Autodesk Inventor part; units mm, degrees
ref_plane "YZ Plane" through (0, 0, 0) normal (1, 0, 0) x (0, 1, 0)
ref_plane "XZ Plane" through (0, 0, 0) normal (0, 1, 0) x (-1, 0, 0)
ref_plane "XY Plane" through (0, 0, 0) normal (0, 0, 1) x (1, 0, 0)
sketch "Sketch1" plane through (0, 0, 0) normal (0, 0, 1) x (1, 0, 0)
  line L0 (0, 0) -> (25.4, 0)
  line L1 (25.4, 0) -> (25.4, 50.8)
  line L2 (25.4, 50.8) -> (0, 50.8)
  line L3 (0, 50.8) -> (0, 0)
  dimension "d0" = 25.4
  dimension "d1" = 50.8
extrude "Extrusion1" add sketch "Sketch1" along normal blind 203.2
shell "Shell1" thickness 2.54 removed faces 2 at (8.4667, 33.8667, 0) at (8.4667, 33.8667, 203.2)
sketch "Sketch2" plane through (0, 50.8, 0) normal (0, 1, 0) x (1, 0, 0)
  line L0 (25.4, 0) -> (0, 0)
  line L1 (0, 0) -> (0, -203.2)
  point P0 (12.7, -12.7)
  point P1 (12.7, -38.1)
  point P2 (12.7, -63.5)
  point P3 (12.7, -88.9)
  point P4 (12.7, -114.3)
  point P5 (12.7, -139.7)
  point P6 (12.7, -165.1)
  point P7 (12.7, -190.5)
  point P8 (12.7, -215.9)
  point P9 (12.7, -241.3)
  point P10 (12.7, -266.7)
  point P11 (12.7, -292.1)
  point P12 (12.7, -317.5)
  point P13 (12.7, -342.9)
  point P14 (12.7, -368.3)
  point P15 (12.7, -393.7)
  point P16 (12.7, -419.1)
  point P17 (12.7, -444.5)
  point P18 (12.7, -469.9)
  point P19 (12.7, -495.3)
  point P20 (12.7, -520.7)
  point P21 (12.7, -546.1)
  point P22 (12.7, -571.5)
  point P23 (12.7, -596.9)
  point P24 (12.7, -622.3)
  point P25 (12.7, -647.7)
  point P26 (12.7, -673.1)
  point P27 (12.7, -698.5)
  point P28 (12.7, -723.9)
  point P29 (12.7, -749.3)
  point P30 (12.7, -774.7)
  point P31 (12.7, -800.1)
  point P32 (12.7, -825.5)
  point P33 (12.7, -850.9)
  point P34 (12.7, -876.3)
  point P35 (12.7, -901.7)
  point P36 (12.7, -927.1)
  dimension "d5" = 12.7
  dimension "d6" = 12.7
  dimension "d9" = 25.4
hole "Hole1" at (12.7, 50.8, 12.7) at (12.7, 50.8, 38.1) at (12.7, 50.8, 63.5) at (12.7, 50.8, 88.9) at (12.7, 50.8, 114.3) at (12.7, 50.8, 139.7) at (12.7, 50.8, 165.1) at (12.7, 50.8, 190.5) at (12.7, 50.8, 215.9) at (12.7, 50.8, 241.3) at (12.7, 50.8, 266.7) at (12.7, 50.8, 292.1) at (12.7, 50.8, 317.5) at (12.7, 50.8, 342.9) at (12.7, 50.8, 368.3) at (12.7, 50.8, 393.7) at (12.7, 50.8, 419.1) at (12.7, 50.8, 444.5) at (12.7, 50.8, 469.9) at (12.7, 50.8, 495.3) at (12.7, 50.8, 520.7) at (12.7, 50.8, 546.1) at (12.7, 50.8, 571.5) at (12.7, 50.8, 596.9) at (12.7, 50.8, 622.3) at (12.7, 50.8, 647.7) at (12.7, 50.8, 673.1) at (12.7, 50.8, 698.5) at (12.7, 50.8, 723.9) at (12.7, 50.8, 749.3) at (12.7, 50.8, 774.7) at (12.7, 50.8, 800.1) at (12.7, 50.8, 825.5) at (12.7, 50.8, 850.9) at (12.7, 50.8, 876.3) at (12.7, 50.8, 901.7) direction (0, -1, 0) diameter 2.54 depth 50.8 tip angle 118
sketch "Sketch14" plane through (0, 0, 0) normal (-1, 0, 0) x (0, 0, 1)
  circle A0 centre (25.4, 25.4) radius 6.35
  point P0 (0, 0)
hole "Hole6" at (0, 25.4, 25.4) direction (1, 0, 0) diameter 28.575 depth 25.4 tip angle 118
sketch "Sketch15" plane through (25.4, 0, 0) normal (1, 0, 0) x (0, 0, -1)
  circle A0 centre (-177.8, 25.4) radius 20
  point P0 (0, 0)
hole "Hole7" at (25.4, 25.4, 177.8) direction (-1, 0, 0) diameter 28.575 depth 25.4 tip angle 118
sketch "Sketch16" plane through (25.4, 0, 0) normal (1, 0, 0) x (0, 0, -1)
  circle A0 centre (-159.8395, 43.3605) radius 3.3655
  circle A1 centre (-195.7605, 7.4395) radius 3.3655
  circle A2 centre (-195.3, 42.9) radius 3.3655
  circle A3 centre (-160.3, 7.9) radius 3.1115
  point P0 (0, 0)
hole "Hole8" at (25.4, 7.9, 160.3) at (25.4, 43.3605, 159.8395) at (25.4, 42.9, 195.3) at (25.4, 7.4395, 195.7605) direction (-1, 0, 0) diameter 4.4958 depth 25.4 tip angle 118
properties part number "Support Pivs 2522" material "Aluminum 6061"
The listing builds one solid part. Answer for the finished solid, in the listing's coordinates (mm). A direction names the side the tool comes from. Give positions to 0.01 mm unless a question says otherwise; leave off trailing zeros. Order: outer loops, then holes, each group sorted by start corner. A loop starts at its lowest first (then second) coordinate and runs counter-clockwise, first axis right, second up. Notation, with made-up numbers: (-20, 3.5) - (25, 3.5) arc R4 cw to (25, 8.5) - close; hole circle Ø6 at (84, 44.25). An arc over 180 degrees is marked (long way). Use one line per item in the form item = value. Start each with the question number.
(1) A cutting plane is placed at B-B, the plane y = 35.5. Write down the section's boundary in (x, z).
(2) A cutting plane is placed at A-A, the plane x = 7. Write down the section's boundary in (y, z).
(3) Consider line 1 (Z direction, x = 23.5, y = 25.5); line 2 (Y direction, x = 24.25, z = 25.4); line 3 (Y direction, x = 12.25, z = 148.5). Determine where each line is inside the solid, lowest interval first. Write a range as from..to.
(4) The mould has two halves that part along Y. Classify faces 1 (the flat face through (13, 50.8, 100)), 2 (the flat face through (2, 27, 203.2)), 3 (the flat face through (13, 0, 100)), 4 (the cylindrical face through (1.252, 42.225, 193.156)): released by +Y, released by -Y, zero draft, split by the parting line, or undercut.
(5) A cutting plane is placed at D-D, the plane z = 195.3. Write down the section's boundary in (x, y), then the cut area to 3 significant figures.
(6) A cutting plane is placed at C-C, the plane z = 45. Write down the section's boundary in (x, y).
(7) For faces 5 (the cylindrical face through (24.148, 15.744, 14.87)), 6 (the flat face through (22.86, 25, 100)), determine the directions among +Z, -Z, +X, -X, +Y, -Y from which every point of the face is accessible in a straight line to the end or side of a thin tool.
Ans:
q1.outline = (0, 0) - (2.54, 0) - (2.54, 15.29) - (0, 15.29) - close; (0, 35.51) - (2.54, 35.51) - (2.54, 167.69) - (0, 167.69) - close; (0, 187.91) - (2.54, 187.91) - (2.54, 203.2) - (0, 203.2) - close; (22.86, 0) - (25.4, 0) - (25.4, 15.29) - (22.86, 15.29) - close; (22.86, 35.51) - (25.4, 35.51) - (25.4, 167.69) - (22.86, 167.69) - close; (22.86, 187.91) - (25.4, 187.91) - (25.4, 203.2) - (22.86, 203.2) - close
q2.outline = (0, 0) - (2.54, 0) - (2.54, 203.2) - (0, 203.2) - close; (48.26, 0) - (50.8, 0) - (50.8, 203.2) - (48.26, 203.2) - close
q3.line_1 = 0..11.11, 39.69..163.51, 192.09..203.2
q3.line_2 = 0..11.11, 39.69..50.8
q3.line_3 = 0..2.54, 48.26..50.8
q4.face_1 = released by +Y
q4.face_2 = zero draft
q4.face_3 = released by -Y
q4.face_4 = undercut
q5.outline = (0, 0) - (25.4, 0) - (25.4, 5.24) - (22.86, 5.24) - (22.86, 2.54) - (2.54, 2.54) - (2.54, 5.24) - (0, 5.24) - close; (0, 9.64) - (2.54, 9.64) - (2.54, 40.65) - (0, 40.65) - close; (0, 45.15) - (2.54, 45.15) - (2.54, 48.26) - (22.86, 48.26) - (22.86, 45.15) - (25.4, 45.15) - (25.4, 50.8) - (0, 50.8) - close; (22.86, 9.64) - (25.4, 9.64) - (25.4, 40.65) - (22.86, 40.65) - close
q5.area = 316 mm^2
q6.outline = (0, 0) - (25.4, 0) - (25.4, 50.8) - (0, 50.8) - close; hole (2.54, 2.54) - (22.86, 2.54) - (22.86, 48.26) - (2.54, 48.26) - close
q7.face_5 = +X, -X
q7.face_6 = +Z, -Z
